Input: part model. Units: mm. Frame: model coordinates. A direction names the side the tool comes from. Round coordinates to 2 decimals unless told otherwise and drop trailing zeros. Loops run counter-clockwise (first coordinate to the right, second up) from the corner with the lowest first, then second, coordinate; pieces in that order, holes last. Notation, with made-up numbers: M -9,-24 L 2,-24 A20 ccw 2,-15 Z; hole C 49,-6.75 d3. An arc over 180 degrees is marked long. Put each result on its own line as item: value. Start each with the question number.
1) Line query: probe 1 along X at (y, z) = (59, 5.75); probe 2 along X at (y, z) = (15, -17.5); probe 3 along Z at (x, y) = (-16, 38). Output: solid intervals per line, ascending.
2) Section C-C on z = -11.75. Output: boundary loops of the cut face in (x, y).
3) Section B-B on y = 18. Output: boundary loops of the cut face in (x, z), plus the area to 3 significant figures.
4) Section A-A on z = 21.2. Output: boundary loops of the cut face in (x, y).
5) Section D-D on z = 5.75. Output: boundary loops of the cut face in (x, y).
6) Pin query (flat end, axial travel): pin 1 (6 mm diameter, centred on y = 52, z = -23.5, fed in from +X); pin 2 (1.5 mm diameter, centred on x = -20, z = 6, fed in from +Y); pin 3 (5.5 mm diameter, centred on x = 12, z = 4.5, fed in from +Y); pin 4 (3.5 mm diameter, centred on x = 17, y = 38.5, fed in from -Z). Return the tip coordinate at first contact, or that it passes through.
7) Reachability of faces 1 (the face through (13.84, 58.82, 34.17)), 2 (the face through (16, 30, -2.5)), 3 (the face through (-14.524, 30, -13)), 4 (the face through (-23, 30, -2.5)), 5 (the face through (-5, 28, 0)) from +Z, -Z, +X, -X, +Y, -Y: full face, straight path, thin tool, end or side. Return the list, or none.
8) Draft query along X for faces 6 (the face through (6.476, 30, -25)), 7 (the face through (-18.524, 30, -13)), 8 (the face through (-16.552, 39.548, -10.331)), 9 (the face through (14.43, 58.82, 7.63)). Return one class per face: +X half, -X half, draft (parallel to the pull), parting line (faces both ways), or undercut.
from build123d import *

# Parameters (mm, degrees)
SKETCH1_W                                           = 45
SKETCH1_H                                           = 60
BOSS_EXTRUDE1_DEPTH                                 = 23.5
SKETCH2_W                                           = 45
SKETCH2_H                                           = 4
BOSS_EXTRUDE2_DEPTH                                 = 45
SKETCH4_W                                           = 21
SKETCH4_H                                           = 21
CUT_EXTRUDE1_DEPTH                                  = 80.552141881
CUT_EXTRUDE2_REACH                                  = 81.552
SKETCH5_R                                           = 12.5
SKETCH13_W                                          = 21
SKETCH13_H                                          = 60
CUT_EXTRUDE3_DEPTH                                  = 8
SKETCH14_W                                          = 21
SKETCH14_H                                          = 60
CUT_EXTRUDE4_DEPTH                                  = 8
SKETCH22_W                                          = 4
SKETCH22_H                                          = 60
BOSS_EXTRUDE6_DEPTH                                 = 25
CBORE_FOR_M3_PAN_HEAD_MACHINE_SCREW1_D              = 3.4
CBORE_FOR_M3_PAN_HEAD_MACHINE_SCREW1_DEPTH          = 4.001
CBORE_FOR_M3_PAN_HEAD_MACHINE_SCREW1_CBORE_D        = 7
CBORE_FOR_M3_PAN_HEAD_MACHINE_SCREW1_CBORE_DEPTH    = 2.4
CBORE_FOR_M3_PAN_HEAD_MACHINE_SCREW1_ON_D           = 3.4
CBORE_FOR_M3_PAN_HEAD_MACHINE_SCREW1_ON_DEPTH       = 4.001
CBORE_FOR_M3_PAN_HEAD_MACHINE_SCREW1_ON_CBORE_D     = 7
CBORE_FOR_M3_PAN_HEAD_MACHINE_SCREW1_ON_CBORE_DEPTH = 2.4
SKETCH16_R                                          = 2.1
CUT_EXTRUDE5_DEPTH                                  = 86.564303305
BOSS_EXTRUDE5_DEPTH                                 = 3
BOSS_EXTRUDE5_DEPTH_BACK                            = 1
SKETCH21_W                                          = 47.5
SKETCH21_H                                          = 60


with BuildPart() as part:
    # Sketch1 → Boss-Extrude1 (new body)
    with BuildSketch(Plane.XY):
        with Locations((-4.024390244, 30)):
            Rectangle(SKETCH1_W, SKETCH1_H)
    extrude(amount=-BOSS_EXTRUDE1_DEPTH)

    # Sketch2 → Boss-Extrude2 (add)
    with BuildSketch(Plane.XY):
        with Locations((-4.024390244, 58)):
            Rectangle(SKETCH2_W, SKETCH2_H)
    extrude(amount=BOSS_EXTRUDE2_DEPTH)

    # Sketch4 → Cut-Extrude1 (cut, through all)
    with BuildSketch(Plane.XZ):
        with Locations((-4.024390244, -13)):
            Rectangle(SKETCH4_W, SKETCH4_H)
    extrude(amount=-CUT_EXTRUDE1_DEPTH, mode=Mode.SUBTRACT)

    # Sketch5 → Cut-Extrude2 (cut, up to next)
    with BuildSketch(Plane(origin=(0, 60, 0), x_dir=(1, 0, 0), z_dir=(0, 1, 0)), mode=Mode.PRIVATE) as cut_extrude2_sk1:
        with Locations(Location((-3.724390244, -21.2, 0), (0, 0, 270))):
            Circle(SKETCH5_R)
    cut_extrude2_tool1 = extrude(cut_extrude2_sk1.sketch, amount=-CUT_EXTRUDE2_REACH, mode=Mode.PRIVATE) & part.part
    add(cut_extrude2_tool1.solids().sort_by_distance((-3.72439, 60, 21.2))[0], mode=Mode.SUBTRACT)

    # Sketch13 → Cut-Extrude3 (cut)
    with BuildSketch(Plane(origin=(18.475609756, 0, 0), x_dir=(0, 0, -1), z_dir=(1, 0, 0))):
        with Locations((13, 30)):
            Rectangle(SKETCH13_W, SKETCH13_H)
    extrude(amount=-CUT_EXTRUDE3_DEPTH, mode=Mode.SUBTRACT)

    # Sketch14 → Cut-Extrude4 (cut)
    with BuildSketch(Plane.ZY.offset(26.524390244)):
        with Locations((-13, 30)):
            Rectangle(SKETCH14_W, SKETCH14_H)
    extrude(amount=-CUT_EXTRUDE4_DEPTH, mode=Mode.SUBTRACT)

    # Sketch22 → Boss-Extrude6 (add)
    with BuildSketch(Plane(origin=(0, 0, -23.5), x_dir=(-1, 0, 0), z_dir=(0, 0, -1))):
        with Locations((-8.475609756, 30)):
            Rectangle(SKETCH22_W, SKETCH22_H)
    extrude(amount=BOSS_EXTRUDE6_DEPTH)

    # CBORE for M3 Pan Head Machine Screw1
    with Locations(Plane(origin=(-19.524390244, 60, 5.75), x_dir=(0, 0, 1), z_dir=(0, 1, 0))):
        with Locations((0, 0), (31, 31), (31, 0), (0, 31)):
            CounterBoreHole(CBORE_FOR_M3_PAN_HEAD_MACHINE_SCREW1_D / 2, CBORE_FOR_M3_PAN_HEAD_MACHINE_SCREW1_CBORE_D / 2, CBORE_FOR_M3_PAN_HEAD_MACHINE_SCREW1_CBORE_DEPTH, depth=CBORE_FOR_M3_PAN_HEAD_MACHINE_SCREW1_DEPTH)

    # CBORE for M3 Pan Head Machine Screw1 on
    with Locations(Plane(origin=(-42.937475152, 0, 35.255713856), x_dir=(0, 0, 1), z_dir=(0, 1, 0))):
        with Locations((0, 0)):
            CounterBoreHole(CBORE_FOR_M3_PAN_HEAD_MACHINE_SCREW1_ON_D / 2, CBORE_FOR_M3_PAN_HEAD_MACHINE_SCREW1_ON_CBORE_D / 2, CBORE_FOR_M3_PAN_HEAD_MACHINE_SCREW1_ON_CBORE_DEPTH, depth=CBORE_FOR_M3_PAN_HEAD_MACHINE_SCREW1_ON_DEPTH)

    # Sketch16 → Cut-Extrude5 (cut, through all)
    with BuildSketch(Plane.ZY.offset(18.524390244)):
        with Locations(Location((-11.75, 38, 0), (0, 0, 270))):
            Circle(SKETCH16_R)
        with Locations((-11.75, 18)):
            Circle(SKETCH16_R)
    extrude(amount=-CUT_EXTRUDE5_DEPTH, mode=Mode.SUBTRACT)

    # Sketch21 → Boss-Extrude5 (add, two sides: drawn at the far end of the back side and taken through both)
    with BuildSketch(Plane(origin=(18.475609756, 0, 0), x_dir=(0, 0, -1), z_dir=(1, 0, 0)).offset(-BOSS_EXTRUDE5_DEPTH_BACK)):
        with Locations((-21.25, 30)):
            Rectangle(SKETCH21_W, SKETCH21_H)
    extrude(amount=BOSS_EXTRUDE5_DEPTH + BOSS_EXTRUDE5_DEPTH_BACK)


solid = part.part
Geometry results:
1. probe 1: x = -26.52 to -23.02, -16.02 to 7.98, 14.98 to 21.48
1. probe 2: x = -18.52 to -14.52, 6.48 to 10.48
1. probe 3: z = -23.5 to -13.85, -9.65 to 0
2. outline: M -18.52,0 L -14.52,0 L -14.52,15.9 L -18.52,15.9 Z; M -18.52,20.1 L -14.52,20.1 L -14.52,35.9 L -18.52,35.9 Z; M -18.52,40.1 L -14.52,40.1 L -14.52,60 L -18.52,60 Z; M 6.48,0 L 10.48,0 L 10.48,15.9 L 6.48,15.9 Z; M 6.48,20.1 L 10.48,20.1 L 10.48,35.9 L 6.48,35.9 Z; M 6.48,40.1 L 10.48,40.1 L 10.48,60 L 6.48,60 Z
3. outline: M -26.52,-2.5 L -18.52,-2.5 L -18.52,-9.65 L -14.52,-9.65 L -14.52,-2.5 L 6.48,-2.5 L 6.48,-9.65 L 10.48,-9.65 L 10.48,-2.5 L 21.48,-2.5 L 21.48,45 L 17.48,45 L 17.48,0 L -26.52,0 Z; M -18.52,-23.5 L -14.52,-23.5 L -14.52,-13.85 L -18.52,-13.85 Z; M 6.48,-48.5 L 10.48,-48.5 L 10.48,-13.85 L 6.48,-13.85 Z
3. area: 534 mm²
4. outline: M -26.52,56 L -16.22,56 L -16.22,60 L -26.52,60 Z; M 8.78,56 L 17.48,56 L 17.48,0 L 21.48,0 L 21.48,60 L 8.78,60 Z
5. outline: M -26.52,56 L -21.22,56 L -21.22,57.6 L -23.02,57.6 L -23.02,60 L -26.52,60 Z; M -17.82,56 L 9.78,56 L 9.78,57.6 L 7.98,57.6 L 7.98,60 L -16.02,60 L -16.02,57.6 L -17.82,57.6 Z; M 13.18,56 L 17.48,56 L 17.48,0 L 21.48,0 L 21.48,60 L 14.98,60 L 14.98,57.6 L 13.18,57.6 Z
6. pin 1: stops at x = 10.48
6. pin 2: passes through
6. pin 3: stops at y = 60
6. pin 4: stops at z = -2.5
7. face 1: +Y
7. face 2: -Z, +X, +Y, -Y
7. face 3: -Z, +Y, -Y
7. face 4: -Z, -X, +Y, -Y
7. face 5: +Z, -X, -Y
8. face 6: undercut
8. face 7: -X half
8. face 8: draft
8. face 9: undercut
